Geometry check sheet. Reference: the model listing, model coordinates, mm. A direction names the side the tool comes from. Coordinates: 2 decimals unless noted, no trailing zeros. Loops run counter-clockwise (first coordinate to the right, second up) from the corner with the lowest first, then second, coordinate; pieces in that order, holes last. Notation, with made-up numbers: M -14.5,58 L 30.5,58 A21 cw 30.5,86 Z; hole C 19,34 d11. An arc over 180 degrees is marked long. One line per question, with ' | ' between items. Start each with the question number.
Autodesk Inventor part; units mm, degrees
ref_plane "YZ Plane" through (0, 0, 0) normal (1, 0, 0) x (0, 1, 0)
ref_plane "XZ Plane" through (0, 0, 0) normal (0, 1, 0) x (-1, 0, 0)
ref_plane "XY Plane" through (0, 0, 0) normal (0, 0, 1) x (1, 0, 0)
sketch "Sketch1" plane through (0, 0, 0) normal (0, 0, 1) x (1, 0, 0)
  line L0 (0, 0) -> (0, 12.7) construction
  line L1 (0, 0) -> (0, -12.7) construction
  circle A0 centre (0, 12.7) radius 1.27
  circle A1 centre (0, -12.7) radius 1.27
  arc A2 (12.7, 12.7) -> (-12.7, 12.7) centre (0, 12.7) ccw
  arc A3 (-12.7, -12.7) -> (12.7, -12.7) centre (0, -12.7) ccw
  line L2 (-12.7, -12.7) -> (-12.7, 12.7)
  line L3 (12.7, 12.7) -> (12.7, -12.7)
  circle A4 centre (0, 0) radius 6.477
  circle A5 centre (0, 0) radius 5.08
  dimension "d0" = 12.7
  dimension "d1" = 12.7
  dimension "d2" = 2.54
  dimension "d3" = 2.54
  dimension "d4" = 25.4
  dimension "d5" = 25.4
  dimension "d6" = 12.954
  dimension "d7" = 10.16
extrude "Extrusion1" add sketch "Sketch1" along normal blind 2.54 contours L3 A3 L2 A2 | A4
extrude "Extrusion2" add sketch "Sketch1" against normal blind 2.54 contours A4
properties part number "bearing_bracket_cover_3DPrint"
1. Tool access check on faces 4 (the cylindrical face through (-0.17, -13.96, 1.25)), 5 (the cylindrical face through (-1.404, -6.323, -1.252)). Record the directions out of +Z, -Z, +X, -X, +Y, -Y that give a thin tool (end or side, any length) a straight path to the whole face; none if there is none.
2. Sectioned sample at A-A (y = 0). Record the cut outline in (x, z), and give its area (3 significant figures).
3. Sectioned sample at B-B (x = 0). Record the cut outline in (y, z).
4. Sectioned sample at D-D (x = 4). Record the cut outline in (y, z).
5. Depth check by flat-ended pin: pin 1 Ø1.5 at (x, z) = (5.5, 0.5) entering from -Y; pin 2 Ø2 at (x, y) = (-10, -17) entering from -Z. Enter the tip coordinate at first touch or a pass-through.
6. Thickness scan on line 1 (Y direction, x = 0, z = 1.8); line 2 (Z direction, x = 9.25, y = -6); line 3 (X direction, y = 13, z = 1.85). Record the ranges inside material, lowest first.
7. Sectioned sample at C-C (z = 0.7). Record the cut outline in (x, y), and give its area (3 significant figures).
8. Draft check along X on faces 1 (the cylindrical face through (-0.661, 5.037, 0.036)), 2 (the flat face through (-0.2, -5.3, 2.54)), 3 (the flat face through (-12.7, 0, 1)). Enter one of: +X half, -X half, draft (parallel to the pull), parting line (faces both ways), or undercut.
Result:
1) face 4: +Z, -Z | face 5: -Z
2) outline: M -12.7,0 L -6.48,0 L -6.48,-2.54 L -5.08,-2.54 L -5.08,2.54 L -12.7,2.54 Z; M 5.08,-2.54 L 6.48,-2.54 L 6.48,0 L 12.7,0 L 12.7,2.54 L 5.08,2.54 Z | area: 45.8 mm2
3) outline: M -25.4,0 L -13.97,0 L -13.97,2.54 L -25.4,2.54 Z; M -11.43,0 L -6.48,0 L -6.48,-2.54 L -5.08,-2.54 L -5.08,2.54 L -11.43,2.54 Z; M 5.08,-2.54 L 6.48,-2.54 L 6.48,0 L 11.43,0 L 11.43,2.54 L 5.08,2.54 Z; M 13.97,0 L 25.4,0 L 25.4,2.54 L 13.97,2.54 Z
4) outline: M -24.75,0 L -5.09,0 L -5.09,-2.54 L -3.13,-2.54 L -3.13,2.54 L -24.75,2.54 Z; M 3.13,-2.54 L 5.09,-2.54 L 5.09,0 L 24.75,0 L 24.75,2.54 L 3.13,2.54 Z
5) pin 1: stops at y = -24.48 | pin 2: stops at z = 0
6) line 1: y = -25.4 to -13.97, -11.43 to -5.08, 5.08 to 11.43, 13.97 to 25.4 | line 2: z = 0 to 2.54 | line 3: x = -12.7 to -1.23, 1.23 to 12.7
7) outline: M -12.7,-12.7 A12.7 ccw 12.7,-12.7 L 12.7,12.7 A12.7 ccw -12.7,12.7 Z; hole C 0,0 d10.16; hole C 0,-12.7 d2.54; hole C 0,12.7 d2.54 | area: 1,060 mm2
8) face 1: undercut | face 2: draft | face 3: -X half
